Source: CAD feature listing. Evaluate the final solid. Frame: model axes, mm. A direction names the side the tool comes from. Give positions to 0.01 mm unless a question says otherwise; leave off trailing zeros. Write each loop counter-clockwise with the first axis right and the second up, starting at its lowest first coordinate (ties: lowest second). Pieces come first, ordered by that corner, then holes. Notation, with made-up numbers: M -31,84 L 5,84 A25 cw 5,108 Z; hole C 27,66 d8. An arc over 180 degrees is marked long. Return JSON: item names as keys, results as strings.
```python
from build123d import *

# Parameters (mm, degrees)
F1_DEPTH = 75
F3_DEPTH = 200
F4_W     = 37
F4_H     = 40
F4_W_2   = 33
F5_DEPTH = 6.5


# Not quite as in the source:
# - a feature names something its author has since deleted; it is built from what else it names


with BuildPart() as f1:
    # F0 (on Front) → F1 (new body, symmetric)
    with BuildSketch(Plane.XZ):
        with BuildLine():
            Line((-67, 35), (70, 35))
            ThreePointArc((70, 35), (91.2132034356, 26.2132034356), (100, 5))
            Line((100, 5), (100, -5))
            ThreePointArc((100, -5), (91.2132034356, -26.2132034356), (70, -35))
            Line((70, -35), (-100, -35))
            Line((-100, -35), (-100, -38))
            Line((-100, -38), (70, -38))
            ThreePointArc((70, -38), (93.3345237792, -28.3345237792), (103, -5))
            Line((103, -5), (103, 5))
            ThreePointArc((103, 5), (93.3345237792, 28.3345237792), (70, 38))
            Line((70, 38), (-67, 38))
            ThreePointArc((-67, 38), (-88.2132034356, 46.7867965644), (-97, 68))
            Line((-97, 68), (-97, 262))
            ThreePointArc((-97, 262), (-88.2132034356, 283.2132034356), (-67, 292))
            Line((-67, 292), (50, 292))
            Line((50, 292), (50, 295))
            Line((50, 295), (-67, 295))
            ThreePointArc((-67, 295), (-90.3345237792, 285.3345237792), (-100, 262))
            Line((-100, 262), (-100, 68))
            ThreePointArc((-100, 68), (-90.3345237792, 44.6654762208), (-67, 35))
        make_face()
    extrude(amount=F1_DEPTH, both=True)

    # F2 (on face) → F3 (cut)
    with BuildSketch(Plane(origin=(-100, 0, 0), x_dir=(0, -1, 0), z_dir=(-1, 0, 0))):
        Polygon((-32.268722467, 262), (-75, 262), (-75, 68), align=None)
        Polygon((-75, 295), (-75, 262), (-32.268722467, 262), (-25, 295), align=None)
        Polygon((25, 295), (32.268722467, 262), (75, 262), (75, 295), align=None)
        Polygon((32.268722467, 262), (75, 68), (75, 262), align=None)
    extrude(amount=-F3_DEPTH, mode=Mode.SUBTRACT)

    # F4 (on face) → F5 (cut, symmetric)
    with BuildSketch(Plane.XY.offset(38)):
        with Locations((51.5, -20)):
            Rectangle(F4_W, F4_H)
        with Locations((86.5, -20)):
            Rectangle(F4_W_2, F4_H)
        with Locations((86.5, 20)):
            Rectangle(F4_W_2, F4_H)
        with Locations((51.5, 20)):
            Rectangle(F4_W, F4_H)
    extrude(amount=F5_DEPTH, both=True, mode=Mode.SUBTRACT)


solid = f1.part
```
1) Draft query along Y for faces 4 (the face through (-9, 0, 292)), 5 (the face through (61, -40, 36)), 6 (the face through (1, -75, -36)). Return one class per face: released by +Y, released by -Y, zero draft, split by the parting line, or undercut.
Numbers:
{"face 4": "zero draft", "face 5": "undercut", "face 6": "released by -Y"}
2) Cut plane D-D, the plane x = 64.5. Return the cut outline in (y, z), then the cut area to 3 significant figures.
Numbers:
{"outline": "M -75,-38 L 75,-38 L 75,-35 L -75,-35 Z; M -75,35 L -40,35 L -40,38 L -75,38 Z; M 40,35 L 75,35 L 75,38 L 40,38 Z", "area": "660 mm²"}
3) Cut plane A-A, the plane y = -3. Return the cut outline in (x, z), then the cut area to 3 significant figures.
Numbers:
{"outline": "M -100,-38 L 70,-38 A33 ccw 103,-5 L 103,5 A33 ccw 89.67,31.5 L 84.06,31.5 A30 cw 100,5 L 100,-5 A30 cw 70,-35 L -100,-35 Z; M -100,68 A33 ccw -67,35 L 33,35 L 33,38 L -67,38 A30 cw -97,68 L -97,262 A30 cw -67,292 L 50,292 L 50,295 L -67,295 A33 ccw -100,262 Z", "area": "2,310 mm²"}
4) Set-up query: faces 1 (the face through (-88.445, -0.452, 282.979)), 2 (the face through (62, 40, 36)), 3 (the face through (94.38, -1.05, 22.48)). Return all of +Z, -Z, +X, -X, +Y, -Y with unobstructed straight access to the full face (end or side cutting, diameter ignored); none if empty.
Numbers:
{"face 1": "+X, +Y, -Y", "face 2": "+Z, +X", "face 3": "-X, +Y, -Y"}
5) Cut plane B-B, the plane x = -43.5. Return the cut outline in (y, z), then the cut area to 3 significant figures.
Numbers:
{"outline": "M -75,-38 L 75,-38 L 75,-35 L -75,-35 Z; M -75,35 L 75,35 L 75,38 L -75,38 Z; M -25.66,292 L 25.66,292 L 25,295 L -25,295 Z", "area": "1,050 mm²"}
6) Cut plane C-C, the plane y = 48. Return the cut outline in (x, z), then the cut area to 3 significant figures.
Numbers:
{"outline": "M -100,-38 L 70,-38 A33 ccw 103,-5 L 103,5 A33 ccw 70,38 L -67,38 A30 cw -97,68 L -97,190.58 L -100,190.58 L -100,68 A33 ccw -67,35 L 70,35 A30 cw 100,5 L 100,-5 A30 cw 70,-35 L -100,-35 Z", "area": "1,760 mm²"}
7) Contact query for flat-ended pins moving along their axis: pin 1 Ø3 at (x, y) = (86, 15.5) entering from +Z; pin 2 Ø1.5 at (y, z) = (8.5, 36.5) entering from +X; pin 3 Ø5 at (y, z) = (35, -1.5) entering from -X. Output: stop coordinate, or through.
Numbers:
{"pin 1": "stops at z = 31.5", "pin 2": "stops at x = 33", "pin 3": "stops at x = 100"}
8) Line query: line 1 (Z direction, x = 2, y = -6.5); line 2 (Z direction, x = -8.5, y = -32.5); line 3 (X direction, y = 15.5, z = 77.5). Output: solid intervals per line, ascending. Write a range as [from, to].
Numbers:
{"line 1": "z = [-38, -35], [35, 38], [292, 295]", "line 2": "z = [-38, -35], [35, 38]", "line 3": "x = [-100, -97]"}
